The listing builds one solid part. Answer for the finished solid, in the listing's coordinates (mm). Face numbers are marked on the shaded views. Round coordinates to 2 decimals unless told otherwise and drop trailing zeros. Loops run counter-clockwise (first coordinate to the right, second up) from the corner with the lowest first, then second, coordinate; pieces in that order, holes last. Notation, with made-up numbers: (24, 55) -> (63, 55) arc R34 ccw to (63, 87) -> close; hole circle Ø9 at (-3.5, 33.5). An arc over 180 degrees is marked (long way). Use a Markdown table: item, result. Add a question column.
Q1. Section D-D on y = 12 is taken. Give the vertices of the cut face in (x, z), then the cut area to 3 significant figures.
Q2. Section A-A on z = 5.25 is taken. Give the vertices of the cut face in (x, y).
Q3. Given pin 1 Ø1.5 at (x, z) = (20.5, 3) entering from -Y; pin 2 Ø1.5 at (x, z) = (-4, 4.5) entering from +Y, each flat-ended and moving along its own axis, determine where each tip first touches the part or whether it passes through.
Q4. Section B-B on x = 1 is taken. Give the vertices of the cut face in (y, z).
Q5. Consider line 1 (Z direction, x = 11, y = -4.5); line 2 (Y direction, x = 25, z = 2); line 3 (Y direction, x = -21, z = 2.75). Determine where each line is inside the solid, lowest interval first.
Q6. Section C-C on y = 2 is taken. Give the vertices of the cut face in (x, z), then the cut area to 3 significant figures.
Q7. For a pull along Y with two mould halves and no side action, classify the marked faces 1, 2, 3 and 4 as released by +Y, released by -Y, zero draft, split by the parting line, or undercut.
from build123d import *

# Parameters (mm, degrees)
BOSS_EXTRUDE1_DEPTH = 6
BOSS_EXTRUDE2_DEPTH = 0.5


with BuildPart() as part:
    # Sketch1 → Boss-Extrude1 (new body)
    with BuildSketch(Plane.XY):
        Polygon((27.53269207, 15.896007178), (0, 31.792014357), (-27.53269207, 15.896007178), (-27.53269207, -15.896007178), (0, -31.792014357), (27.53269207, -15.896007178), align=None)
    extrude(amount=BOSS_EXTRUDE1_DEPTH)

    # Sketch1<3> → Boss-Extrude2 (add)
    with BuildSketch(Plane.XY):
        Polygon((26.666666667, 15.396007178), (0, 30.792014357), (-26.666666667, 15.396007178), (-26.666666667, -15.396007178), (0, -30.792014357), (26.666666667, -15.396007178), align=None)
        Polygon((12.028130608, 0.833333333), (7.024428275, 0.833333333), (14.24130664, 13.333333333), (18.667658704, 5.666666667), (4.426352064, -19), (-4.426352064, -19), (-18.667658704, 5.666666667), (-14.24130664, 13.333333333), (-7.024428275, 0.833333333), (-12.028130608, 0.833333333), (-11.065880159, -0.833333333), (-6.062177826, -0.833333333), (0, -11.333333333), (6.062177826, -0.833333333), (11.065880159, -0.833333333), align=None, mode=Mode.SUBTRACT)
        Polygon((-15.396007178, 13.333333333), (-19.245008973, 6.666666667), (-23.094010768, 13.333333333), align=None, mode=Mode.SUBTRACT)
        Polygon((0, -9.333333333), (-13.086606102, 13.333333333), (13.086606102, 13.333333333), align=None, mode=Mode.SUBTRACT)
        Polygon((23.094010768, 13.333333333), (19.245008973, 6.666666667), (15.396007178, 13.333333333), align=None, mode=Mode.SUBTRACT)
    extrude(amount=-BOSS_EXTRUDE2_DEPTH)


solid = part.part
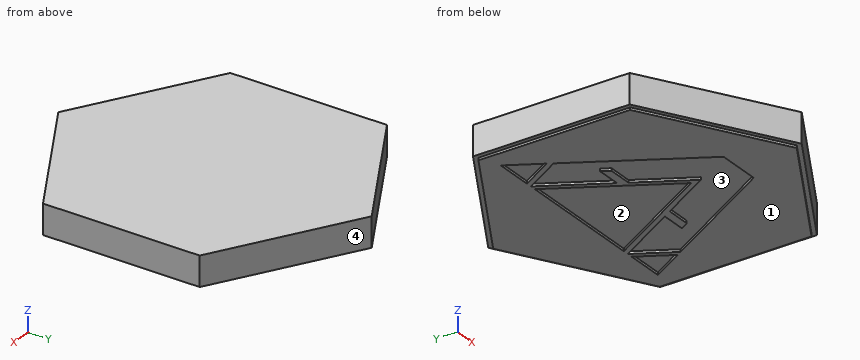
Checked values:
| question | item | result |
|---|---|---|
| 1 | outline | (-27.53, 0) -> (-26.67, 0) -> (-26.67, -0.5) -> (-22.32, -0.5) -> (-22.32, 0) -> (-16.17, 0) -> (-16.17, -0.5) -> (-15.01, -0.5) -> (-15.01, 0) -> (-13.47, 0) -> (-13.47, -0.5) -> (-12.32, -0.5) -> (-12.32, 0) -> (12.32, 0) -> (12.32, -0.5) -> (13.47, -0.5) -> (13.47, 0) -> (15.01, 0) -> (15.01, -0.5) -> (16.17, -0.5) -> (16.17, 0) -> (22.32, 0) -> (22.32, -0.5) -> (26.67, -0.5) -> (26.67, 0) -> (27.53, 0) -> (27.53, 6) -> (-27.53, 6) -> close |
| 1 | area | 337 mm2 |
| 2 | outline | (-27.53, -15.9) -> (0, -31.79) -> (27.53, -15.9) -> (27.53, 15.9) -> (0, 31.79) -> (-27.53, 15.9) -> close |
| 3 | pin 1 | stops at y = -20.39 |
| 3 | pin 2 | stops at y = 29.92 |
| 4 | outline | (-31.21, 0) -> (-30.21, 0) -> (-30.21, -0.5) -> (-19, -0.5) -> (-19, 0) -> (-9.6, 0) -> (-9.6, -0.5) -> (-7.6, -0.5) -> (-7.6, 0) -> (13.33, 0) -> (13.33, -0.5) -> (30.21, -0.5) -> (30.21, 0) -> (31.21, 0) -> (31.21, 6) -> (-31.21, 6) -> close |
| 5 | line 1 | z = 0 to 6 |
| 5 | line 2 | y = -17.36 to 17.36 |
| 5 | line 3 | y = -19.67 to 19.67 |
| 6 | outline | (-27.53, 0) -> (-26.67, 0) -> (-26.67, -0.5) -> (-16.55, -0.5) -> (-16.55, 0) -> (-7.7, 0) -> (-7.7, -0.5) -> (-6.54, -0.5) -> (-6.54, 0) -> (6.54, 0) -> (6.54, -0.5) -> (7.7, -0.5) -> (7.7, 0) -> (16.55, 0) -> (16.55, -0.5) -> (26.67, -0.5) -> (26.67, 0) -> (27.53, 0) -> (27.53, 6) -> (-27.53, 6) -> close |
| 6 | area | 342 mm2 |
| 7 | face 1 | zero draft |
| 7 | face 2 | undercut |
| 7 | face 3 | undercut |
| 7 | face 4 | released by +Y |
